The listing builds one solid part. Answer for the finished solid, in the listing's coordinates (mm). Round coordinates to 2 decimals unless told otherwise and drop trailing zeros. Order: outer loops, then holes, each group sorted by start corner. A loop starts at its lowest first (then second) coordinate and runs counter-clockwise, first axis right, second up. Notation, with made-up numbers: M 35.5,-13 L 67.5,-13 A21 ccw 67.5,20 Z; hole C 64,28 d7. An arc over 180 degrees is marked long. Put each result on its own line as item: value. Start each with the question number.
1. Consider line 1 (Z direction, x = 263, y = -75.5); line 2 (Y direction, x = 273, z = 210.5); line 3 (Z direction, x = -218, y = -320). Determine where each line is inside the solid, lowest interval first.
2. The part is cut by section A-A (x = -23). Give the vertices of the cut face in (y, z), then the cut area to 3 significant figures.
3. The part is cut by section B-B (y = -173.5). Give the vertices of the cut face in (x, z), then the cut area to 3 significant figures.
4. The part is cut by section C-C (z = 293). Give the vertices of the cut face in (x, y).
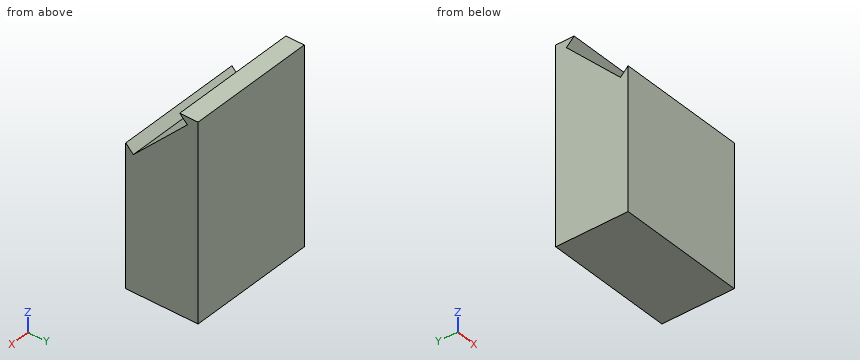
from build123d import *

# Parameters (mm, degrees)
F0_W     = 609.6
F0_H     = 914.4
F1_DEPTH = 340.36
F2_SIZE  = 254
F3_DEPTH = 50.8


with BuildPart() as f1:
    # F0 (on Front) → F1 (new body)
    with BuildSketch(Plane.XZ):
        Rectangle(F0_W, F0_H)
    extrude(amount=F1_DEPTH)

    # F2
    f2_edges = [f1.edges().sort_by_distance(p)[0] for p in [
        (0, -340.36, 457.2),
    ]]
    chamfer(f2_edges, length=F2_SIZE)

    # F3 (cut): a face of the model
    f3_faces = [f1.faces().sort_by_distance(p)[0] for p in [
        (0, -213.36, 330.2),
    ]]
    extrude(f3_faces, amount=-F3_DEPTH, mode=Mode.SUBTRACT)


solid = f1.part
Resolved:
1. line 1: -457.2 to 396.22, 446.34 to 457.2
1. line 2: -261.22 to 0
1. line 3: -457.2 to 182.84
2. outline: M -340.36,-457.2 L 0,-457.2 L 0,457.2 L -86.36,457.2 L -50.44,421.28 L -304.44,167.28 L -340.36,203.2 Z
2. area: 261,000 mm2
3. outline: M -304.8,-457.2 L 304.8,-457.2 L 304.8,298.22 L -304.8,298.22 Z
3. area: 461,000 mm2
4. outline: M -304.8,-178.72 L 304.8,-178.72 L 304.8,0 L -304.8,0 Z
